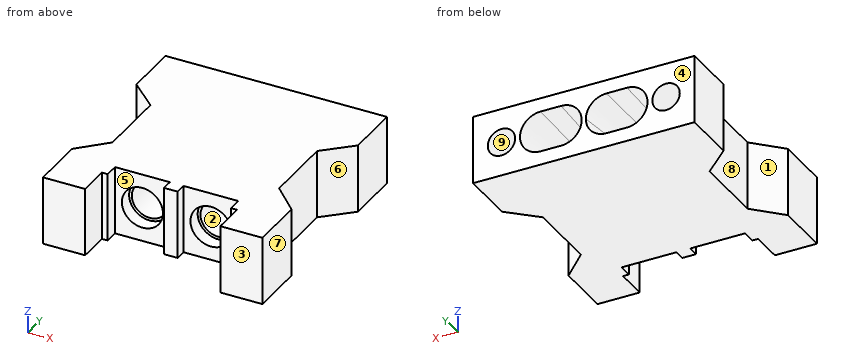
```python
from build123d import *

# Parameters (mm, degrees)
SKETCH072_R            = 2.7
PAD031_DEPTH           = 10
SKETCH069_R            = 2.6
POCKET028_DEPTH        = 10
SKETCH070_R            = 3
POCKET029_DEPTH        = 2
SKETCH073_R            = 2
POCKET030_DEPTH        = 8
CUT003_PLACEMENT_ANGLE = 90


with BuildPart() as loft004:
    # Sketch072 → Loft004 section 0
    with BuildSketch(Plane.XY.offset(20)):
        with Locations((-5, 0)):
            Circle(SKETCH072_R)
    # Sketch071 → Loft004 section 1
    with BuildSketch(Plane.XY.offset(38)):
        with BuildLine():
            ThreePointArc((-6.3, 3), (-9.3, 0), (-6.3, -3))
            Line((-6.3, -3), (-3.3, -3))
            ThreePointArc((-3.3, -3), (-0.3, 0), (-3.3, 3))
            Line((-3.3, 3), (-6.3, 3))
        make_face()
    loft()


with BuildPart() as part_mirroring004:
    # Part__Mirroring004: instance of Loft004
    add(loft004.part.mirror(Plane(origin=(0, 0, 0), x_dir=(0, -1, 0), z_dir=(1, 0, 0))))


with BuildPart() as fusion004:
    # Fusion004 base: copy of Loft004
    add(loft004.part)

    # Fusion004: union Part__Mirroring004
    add(part_mirroring004.part)


with BuildPart() as cut003:
    # Sketch068 → Pad031 (new body)
    with BuildSketch(Plane.XZ):
        Polygon((-16, 4), (-9.85, 4), (-9.85, 7), (-9.85, 8.6), (-9, 8.6), (-9, 10.6), (-1, 10.6), (-1, 9), (1, 9), (1, 10.6), (9, 10.6), (9, 8.6), (9.85, 8.6), (9.85, 7), (9.85, 4), (16, 4), (16, 12), (12.15, 15.85), (12.15, 26.306086), (16.15, 30), (16.15, 38), (-16.15, 38), (-16.15, 30), (-12.15, 26.306086), (-12.15, 15.85), (-16, 12), align=None)
    extrude(amount=PAD031_DEPTH)

    # Sketch069 (on Face7 of Pad031) → Pocket028 (cut)
    with BuildSketch(Plane(origin=(0, 0, 10.6), x_dir=(1, 0, 0), z_dir=(0, 0, -1))):
        with Locations((-5, 5)):
            Circle(SKETCH069_R)
        with Locations((5, 5)):
            Circle(SKETCH069_R)
    extrude(amount=-POCKET028_DEPTH, mode=Mode.SUBTRACT)

    # Sketch070 (on Face11 of Pocket028) → Pocket029 (cut)
    with BuildSketch(Plane(origin=(0, 0, 10.6), x_dir=(1, 0, 0), z_dir=(0, 0, -1))):
        with Locations((-5, 5)):
            Circle(SKETCH070_R)
        with Locations((5, 5)):
            Circle(SKETCH070_R)
    extrude(amount=-POCKET029_DEPTH, mode=Mode.SUBTRACT)

    # Sketch073 (on Face26 of Pocket029) → Pocket030 (cut)
    with BuildSketch(Plane(origin=(0, 0, 38), x_dir=(-1, 0, 0), z_dir=(0, 0, 1))):
        with Locations((-12, 5)):
            Circle(SKETCH073_R)
        with Locations((12, 5)):
            Circle(SKETCH073_R)
    extrude(amount=-POCKET030_DEPTH, mode=Mode.SUBTRACT)


with BuildPart() as cut003_1:
    # Body025 placement: moved
    add(cut003.part.moved(Location((0, 5, 0))))

    # Cut003: cut Fusion004
    add(fusion004.part, mode=Mode.SUBTRACT)


with BuildPart() as cut003_2:
    # Cut003 placement: moved
    add(cut003_1.part.moved(Location((0, -512, 24))).rotate(Axis((0, -512, 24), (-1, 0, 0)), CUT003_PLACEMENT_ANGLE))


solid = cut003_2.part
```
Verification items for the finished model (mm, model axes). Face numbers are marked on the shaded views. A direction names the side the tool comes from. Coordinates: 2 decimals unless noted, no trailing zeros. Loops run counter-clockwise (first coordinate to the right, second up) from the corner with the lowest first, then second, coordinate; pieces in that order, holes last. Notation, with made-up numbers: (-15.75, 69.25) - (-3.75, 69.25) arc R22 cw to (-3.75, 89.25) - close; hole circle Ø7 at (81, 86.25). An arc over 180 degrees is marked (long way). Answer as a JSON object with one key per item and string values.
(1) Cross-section at A-A, the plane y = -502. Record the boundary of the cut face in (x, z).
Response:
{"outline": "(-16, 19) - (-9, 19) - (-9, 29) - (-16, 29) - close; (-1, 19) - (1, 19) - (1, 29) - (-1, 29) - close; (9, 19) - (16, 19) - (16, 29) - (9, 29) - close"}
(2) Cross-section at C-C, the plane z = 25.25. Count the separate pieces of the cut face and the enclosed holes in it, then the cut area to 3 significant figures.
Response:
{"separate pieces": "3", "enclosed holes": "0", "area": "481 mm²"}
(3) Access from +Z, -Z, +X, -X, +Y, -Y to the whole of each face (thin tool, end or side, straight path). Record for the marked faces 5, 6, 7, 8 and 9.
Response:
{"face 5": "+Z, -Z, -Y", "face 6": "+Z, -Z, +X", "face 7": "+Z, -Z, +X, -Y", "face 8": "+Z, -Z, -X", "face 9": "+Y"}
(4) Mould release check, pull along Y, two halves, no side actions. Record for the marked faces 1, 2, 3 and 4: pulls with the +Y half, pulls with the -Y half, needs draft (parallel to the pull), parting line crosses it, or undercut.
Response:
{"face 1": "undercut", "face 2": "needs draft", "face 3": "pulls with the -Y half", "face 4": "pulls with the +Y half"}
(5) Go/stop test with flat-tipped pins: pin 1 Ø0.6 at (y, z) = (-502.5, 26.5) entering from +X; pin 2 Ø2 at (x, z) = (3, 20) entering from -Y; pin 3 Ø3 at (y, z) = (-501.5, 28) entering from -X; pin 4 Ø3 at (x, z) = (-4.5, 24) entering from -Y. Record where each tip stops, or that it passes through.
Response:
{"pin 1": "stops at x = 16", "pin 2": "stops at y = -501.4", "pin 3": "stops at x = -16", "pin 4": "passes through"}
(6) Scan lines: line 1 along X through (y, z) = (-502, 22.25); line 2 along Z through (x, y) = (12, -477.5); line 3 along X through (y, z) = (-504, 20.25). Record each from-to range of solid material in increasing order.
Response:
{"line 1": "x = -16 to -9, -1 to 1, 9 to 16", "line 2": "z = 19 to 22, 26 to 29", "line 3": "x = -16 to -9.85, 9.85 to 16"}
(7) Cross-section at B-B, the plane x = 11. Record the boundary of the cut face in (y, z), then the cut area to 3 significant figures.
Response:
{"outline": "(-508, 19) - (-474, 19) - (-474, 22.27) - (-482, 22.27) - (-482, 25.73) - (-474, 25.73) - (-474, 29) - (-508, 29) - close", "area": "312 mm²"}
